Autodesk Fusion 360 part; units mm, degrees
sketch "Sketch1" plane through (0, 0, 0) normal (0, 0, 1) x (1, 0, 0)
  line L0 (440, 422.75) -> (-440, 422.75)
  line L1 (-440, 422.75) -> (-440, -422.75)
  line L2 (-440, -422.75) -> (440, -422.75)
  line L3 (440, -422.75) -> (440, 422.75)
  line L4 (440, 422.75) -> (-440, -422.75) construction
  line L5 (-440, 422.75) -> (440, -422.75) construction
  line L6 (144, -302.75) -> (-236, -302.75)
  line L7 (-236, -302.75) -> (-236, 342.75)
  line L8 (-236, 342.75) -> (144, 342.75)
  line L9 (144, 342.75) -> (144, -302.75)
  line L10 (-295, 5.75) -> (-375, 5.75) construction
  line L11 (-375, 5.75) -> (-375, 240.75) construction
  line L12 (-375, 240.75) -> (-295, 240.75) construction
  line L13 (-295, 240.75) -> (-295, 5.75) construction
  line L14 (375, 5.75) -> (295, 5.75) construction
  line L15 (295, 5.75) -> (295, 240.75) construction
  line L16 (295, 240.75) -> (375, 240.75) construction
  line L17 (375, 240.75) -> (375, 5.75) construction
  line L18 (-46.5, -422.75) -> (-46.5, 422.75) construction
  line L19 (-91.5, -323.55) -> (-1.5, -323.55) construction
  line L20 (-1.5, -323.55) -> (-1.5, -347.55) construction
  line L21 (-1.5, -347.55) -> (-91.5, -347.55) construction
  line L22 (-91.5, -347.55) -> (-91.5, -323.55) construction
  line L23 (-26.5, -319.5853) -> (-26.5, -354.5853) construction
  line L24 (-66.5, -319.5853) -> (-66.5, -354.5853) construction
  circle A0 centre (-26.5, -323.55) radius 6.35
  circle A1 centre (-26.5, -347.55) radius 6.35
  circle A2 centre (-66.5, -323.55) radius 6.35
  circle A3 centre (-66.5, -347.55) radius 6.35
  circle A4 centre (-91.5, -323.55) radius 7.95
  circle A5 centre (-91.5, -347.55) radius 7.95
  circle A6 centre (-1.5, -323.55) radius 7.95
  circle A7 centre (-1.5, -347.55) radius 7.95
  circle A8 centre (-295, 5.75) radius 9.5
  circle A9 centre (-375, 5.75) radius 9.5
  circle A10 centre (-375, 240.75) radius 9.5
  circle A11 centre (-295, 240.75) radius 9.5
  circle A12 centre (295, 240.75) radius 9.5
  circle A13 centre (375, 240.75) radius 9.5
  circle A14 centre (375, 5.75) radius 9.5
  circle A15 centre (295, 5.75) radius 9.5
  line L25 (100, 370.25) -> (-50, 370.25) construction
  circle A16 centre (-69.5, 370.25) radius 7.95
  circle A17 centre (-23.5, 370.25) radius 7.95
  line L26 (-440, 240.75) -> (440, 240.75) construction
  line L27 (-429, 260) -> (-429, -100) construction
  line L28 (429, 260) -> (429, -90) construction
  circle A18 centre (429, 240.75) radius 3.5
  circle A19 centre (429, 240.75) radius 9.5
  circle A20 centre (429, -34.25) radius 3.5
  circle A21 centre (429, -34.25) radius 9.5
  circle A22 centre (-429, 240.75) radius 3.5
  circle A23 centre (-429, 240.75) radius 9.5
  circle A24 centre (-429, -34.25) radius 3.5
  circle A25 centre (-429, -34.25) radius 9.5
  circle A26 centre (-370, -372.75) radius 1.5
  circle A27 centre (370, -372.75) radius 1.5
  circle A28 centre (-370, 372.75) radius 1.5
  circle A29 centre (370, 372.75) radius 1.5
  circle A30 centre (295, -44.25) radius 1.5
  circle A31 centre (-295, -44.25) radius 1.5
  dimension "d1" = 880
  dimension "d2" = 845.5
  dimension "d3" = 380
  dimension "d4" = 645.5
  dimension "d5" = 120
  dimension "d7" = 80
  dimension "d8" = 235
  dimension "d9" = 235
  dimension "d10" = 80
  dimension "d11" = 65
  dimension "d12" = 65
  dimension "d13" = 182
  dimension "d14" = 182
  dimension "d16" = 90
  dimension "d17" = 24
  dimension "d18" = 45
  dimension "d19" = 40
  dimension "d20" = 12.7
  dimension "d21" = 12.7
  dimension "d22" = 12.7
  dimension "d23" = 12.7
  dimension "d24" = 15.9
  dimension "d25" = 15.9
  dimension "d26" = 15.9
  dimension "d27" = 15.9
  dimension "d29" = 20
  dimension "d30" = 75.2
  dimension "d31" = 19
  dimension "d32" = 19
  dimension "d33" = 19
  dimension "d34" = 19
  dimension "d35" = 19
  dimension "d36" = 19
  dimension "d37" = 19
  dimension "d38" = 19
  dimension "d39" = 52.5
  dimension "d40" = 15.9
  dimension "d41" = 15.9
  dimension "d42" = 23
  dimension "d43" = 23
  dimension "d44" = 11
  dimension "d45" = 11
  dimension "d46" = 7
  dimension "d47" = 19
  dimension "d48" = 7
  dimension "d49" = 19
  dimension "d50" = 275
  dimension "d51" = 7
  dimension "d52" = 19
  dimension "d53" = 7
  dimension "d54" = 275
  dimension "d55" = 19
  dimension "d66" = 296
  dimension "d67" = 486.5
  dimension "d84" = 3
  dimension "d85" = 3
  dimension "d86" = 3
  dimension "d87" = 3
  dimension "d88" = 3
  dimension "d89" = 3
  dimension "d90" = 70
  dimension "d91" = 70
  dimension "d92" = 70
  dimension "d93" = 70
  dimension "d94" = 50
  dimension "d95" = 50
  dimension "d96" = 50
  dimension "d97" = 50
  dimension "d98" = 50
  dimension "d99" = 50
extrude "Extrude1" add sketch "Sketch1" along normal blind 18 contours L0 L1 L2 L3 | A19 | A21 | A23 | A25
extrude "Extrude2" cut sketch "Sketch1" along normal blind 5 contours A19 | A21 | A23 | A25
sketch "Sketch2" plane through (0, 0, 18) normal (0, 0, 1) x (-1, 0, 0)
  circle A0 centre (-429, -240.75) radius 3.5
  circle A1 centre (23.5, -370.25) radius 7.95
  circle A2 centre (-429, 34.25) radius 3.5
  circle A3 centre (69.5, -370.25) radius 7.95
  circle A4 centre (429, -240.75) radius 3.5
  circle A5 centre (429, 34.25) radius 3.5
  circle A6 centre (295, -5.75) radius 9.5
  circle A7 centre (375, -240.75) radius 9.5
  circle A8 centre (295, -240.75) radius 9.5
  circle A9 centre (-295, -240.75) radius 9.5
  circle A10 centre (-375, -240.75) radius 9.5
  circle A11 centre (-375, -5.75) radius 9.5
  circle A12 centre (-295, -5.75) radius 9.5
  circle A13 centre (1.5, 347.55) radius 7.95
  circle A14 centre (1.5, 323.55) radius 7.95
  circle A15 centre (91.5, 347.55) radius 7.95
  circle A16 centre (91.5, 323.55) radius 7.95
  circle A17 centre (66.5, 347.55) radius 6.35
  circle A18 centre (66.5, 323.55) radius 6.35
  circle A19 centre (26.5, 347.55) radius 6.35
  circle A20 centre (26.5, 323.55) radius 6.35
  circle A21 centre (375, -5.75) radius 9.5
  line L0 (236, -342.75) -> (-144, -342.75)
  line L1 (-144, -342.75) -> (-144, 302.75)
  line L2 (-144, 302.75) -> (236, 302.75)
  line L3 (236, 302.75) -> (236, -342.75)
  line L4 (-440, 422.75) -> (-440, -422.75)
  line L5 (-440, -422.75) -> (440, -422.75)
  line L6 (440, -422.75) -> (440, 422.75)
  line L7 (440, 422.75) -> (-440, 422.75)
  line L8 (122, 313.05) -> (-29, 313.05)
  line L9 (-29, 313.05) -> (-29, 358.05)
  line L10 (-29, 358.05) -> (122, 358.05)
  line L11 (122, 358.05) -> (122, 313.05)
  line L12 (1.5, 323.55) -> (-29, 323.55) construction
  line L13 (91.5, 323.55) -> (122, 323.55) construction
  line L14 (91.5, 323.55) -> (91.5, 313.05) construction
  line L15 (91.5, 347.55) -> (91.5, 358.05) construction
  circle A22 centre (429, 34.25) radius 9.5
  circle A23 centre (370, -372.75) radius 1.5
  circle A24 centre (-370, 372.75) radius 1.5
  circle A25 centre (-370, -372.75) radius 1.5
  circle A26 centre (-295, 44.25) radius 1.5
  circle A27 centre (295, 44.25) radius 1.5
  circle A28 centre (370, 372.75) radius 1.5
  dimension "d62" = 151
  dimension "d63" = 45
  dimension "d72" = 46
  dimension "d73" = 65
  dimension "d74" = 11
  dimension "d75" = 80
  dimension "d76" = 40
  dimension "d77" = 65
  dimension "d78" = 80
  dimension "d79" = 380
  dimension "d80" = 645.5
  dimension "d81" = 296
  dimension "d82" = 80
  dimension "d83" = 64.7
extrude "Extrude4" cut sketch "Sketch2" against normal blind 8.5 contours L8 L9 L10 L11
equation "d20 = M5WasherClearance"
equation "d21 = M5WasherClearance"
equation "d22 = M5WasherClearance"
equation "d23 = M5WasherClearance"
equation "d24 = M6WasherClearance"
equation "d25 = M6WasherClearance"
equation "d26 = M6WasherClearance"
equation "d27 = M6WasherClearance"
equation "d31 = CrossDowelClearance"
equation "d32 = CrossDowelClearance"
equation "d33 = CrossDowelClearance"
equation "d34 = CrossDowelClearance"
equation "d35 = CrossDowelClearance"
equation "d36 = CrossDowelClearance"
equation "d37 = CrossDowelClearance"
equation "d38 = CrossDowelClearance"
equation "d40 = M6WasherClearance"
equation "d41 = M6WasherClearance"
equation "d46 = M6ClearHole"
equation "d47 = CrossDowelClearance"
equation "d48 = M6ClearHole"
equation "d49 = CrossDowelClearance"
equation "d51 = M6ClearHole"
equation "d52 = CrossDowelClearance"
equation "d53 = M6ClearHole"
equation "d55 = CrossDowelClearance"
equation "CrossDowelClearance = 19 mm"
equation "M6ClearHole = 7 mm"
equation "M6WasherClearance = 15.9 mm"
equation "M5WasherClearance = 12.7 mm"
equation "d91 = d90"
equation "d92 = d90"
equation "d93 = d90"
equation "d95 = d94"
equation "d96 = d94"
equation "d97 = d94"
equation "d98 = d94"
equation "d99 = d94"
Source: CAD feature listing. Evaluate the final solid. Frame: model axes, mm. A direction names the side the tool comes from. Round coordinates to 2 decimals unless told otherwise and drop trailing zeros. Loops run counter-clockwise (first coordinate to the right, second up) from the corner with the lowest first, then second, coordinate; pieces in that order, holes last. Notation, with made-up numbers: M 80,-16.75 L 89,-16.75 A27 ccw 89,15.25 Z; hole C -13,-27.75 d5. An arc over 180 degrees is marked long. Return JSON: item names as keys, results as strings. Group by question number.
1. Section query B-B on z = 12.5. State how many separate pieces and enclosed holes the cut face has, and give its area (3 significant figures).
2. Mould query, pull axis Y, two halves, no side actions, for faces 4 (the face through (189, 6, 18)), 5 (the face through (-286.224, 244.389, 8.874)), 6 (the face through (-384.49, 5.33, 8.87)). Classes: released by +Y, released by -Y, zero draft, split by the parting line, or undercut.
3. Pin query (flat end, axial travel): pin 1 (9 mm diameter, centred on x = -429, y = 240.75, fed in from +Z); pin 2 (9 mm diameter, centred on x = 429, y = -34.25, fed in from -Z). Return the tip coordinate at first contact, or that it passes through.
4. Reachability of faces 1 (the face through (-45, -336, 9.5)), 2 (the face through (-424.62, 249.18, 2.46)), 3 (the face through (303.776, 9.389, 8.874)) from +Z, -Z, +X, -X, +Y, -Y: full face, straight path, thin tool, end or side. Return the list, or none.
5. Section query A-A on y = -71.5. Output: boundary loops of the cut face in (x, z), and give its area (3 significant figures).
6. Material intervals for line 1 along Y through (x, z) = (429, 8.25); line 2 along Y through (x, z) = (375, 14.25); line 3 along X through (y, z) = (217.5, 6), sorted ascending. Write a range as from..to.
Checks:
{
 "1": {"separate pieces": "1", "enclosed holes": "22", "area": "489,000 mm²"},
 "2": {"face 4": "zero draft", "face 5": "undercut", "face 6": "undercut"},
 "3": {"pin 1": "stops at z = 18", "pin 2": "stops at z = 5"},
 "4": {"face 1": "+Z", "face 2": "-Z", "face 3": "+Z, -Z"},
 "5": {"outline": "M -440,0 L -236,0 L -236,18 L -440,18 Z; M 144,0 L 440,0 L 440,18 L 144,18 Z", "area": "9,000 mm²"},
 "6": {"line 1": "y = -422.75..-37.75, -30.75..237.25, 244.25..422.75", "line 2": "y = -422.75..-3.75, 15.25..231.25, 250.25..422.75", "line 3": "x = -440..-236, 144..440"}
}
